Verification items for this drawing (mm, ordinates from the low corner). A direction names the side the tool comes from. Give positions to 0.01 mm unless a question says otherwise; leave off trailing zeros. Loops run counter-clockwise (first coordinate to the right, second up) from the corner with the lowest first, then second, coordinate; pieces in that order, holes last. Notation, with made-up numbers: (53, 66) -> (95, 66) arc R18 cw to (95, 89) -> close; hole circle Ø3 at (62, -18). An arc over 180 degrees is marked (long way). Use one line per item in the form item = value. Start each with the question number.
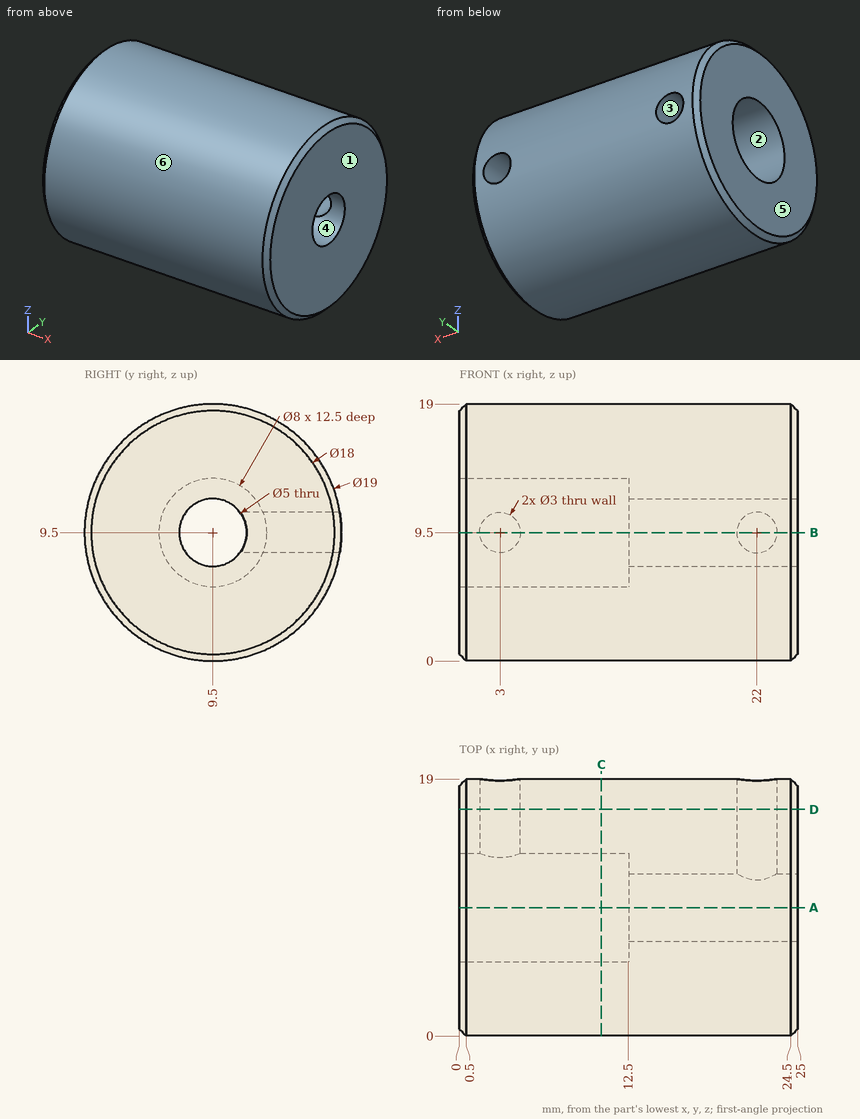
Item 1: Material ranges on line 1 (Z direction, x = 16, y = 9.5); line 2 (Y direction, x = 7, z = 9.75); line 3 (X direction, y = 18, z = 9), recorded low to high.
Item 2: Sectioned sample at B-B, the plane z = 9.5. Enter the section's corners in (x, y).
Item 3: Draft check along Y on the marked faces 4, 5 and 6. Enter one of: +Y half, -Y half, draft (parallel to the pull), parting line (faces both ways), or undercut.
Item 4: Gauge pin test, flat ends, axial feed: pin 1 Ø5 at (x, y) = (4.5, 12.5) entering from +Z; pin 2 Ø6.5 at (y, z) = (9.5, 9.5) entering from -X; pin 3 Ø2.5 at (x, z) = (22, 9.5) entering from +Y. Record the tip position at first contact, or that the pin passes through.
Item 5: Sectioned sample at D-D, the plane y = 16.75. State how many separate pieces and enclosed holes the cut face has, and give its area (3 significant figures).
Item 6: Sectioned sample at C-C, the plane x = 10.5. Enter the section's corners in (y, z), and give its area (3 significant figures).
Item 7: Sectioned sample at A-A, the plane y = 9.5. Enter the section's corners in (x, z), and give its area (3 significant figures).
Item 8: Tool access check on the marked faces 1, 2 and 3. Record the directions out of +Z, -Z, +X, -X, +Y, -Y that give a thin tool (end or side, any length) a straight path to the whole face; none if there is none.
Outcome:
q1.line_1 = 0 to 7, 12 to 19
q1.line_2 = 0 to 5.51, 13.49 to 19
q1.line_3 = 0 to 1.59, 4.41 to 20.59, 23.41 to 25
q2.outline = (0, 0.5) -> (0.5, 0) -> (24.5, 0) -> (25, 0.5) -> (25, 7) -> (12.5, 7) -> (12.5, 5.5) -> (0, 5.5) -> close; (0, 13.5) -> (1.5, 13.5) -> (1.5, 19) -> (0.5, 19) -> (0, 18.5) -> close; (4.5, 13.5) -> (12.5, 13.5) -> (12.5, 12) -> (20.5, 12) -> (20.5, 19) -> (4.5, 19) -> close; (23.5, 12) -> (25, 12) -> (25, 18.5) -> (24.5, 19) -> (23.5, 19) -> close
q3.face_4 = undercut
q3.face_5 = draft
q3.face_6 = parting line
q4.pin_1 = 18.99
q4.pin_2 = 12.5
q4.pin_3 = 7.33
q5.separate_pieces = 1
q5.enclosed_holes = 2
q5.area = 292 mm^2
q6.outline = circle Ø19 at (9.5, 9.5); hole circle Ø8 at (9.5, 9.5)
q6.area = 233 mm^2
q7.outline = (0, 0.5) -> (0.5, 0) -> (24.5, 0) -> (25, 0.5) -> (25, 7) -> (12.5, 7) -> (12.5, 5.5) -> (0, 5.5) -> close; (0, 13.5) -> (12.5, 13.5) -> (12.5, 12) -> (25, 12) -> (25, 18.5) -> (24.5, 19) -> (0.5, 19) -> (0, 18.5) -> close
q7.area = 312 mm^2
q8.face_1 = +Z, -Z, +X, +Y, -Y
q8.face_2 = -X
q8.face_3 = +Y
